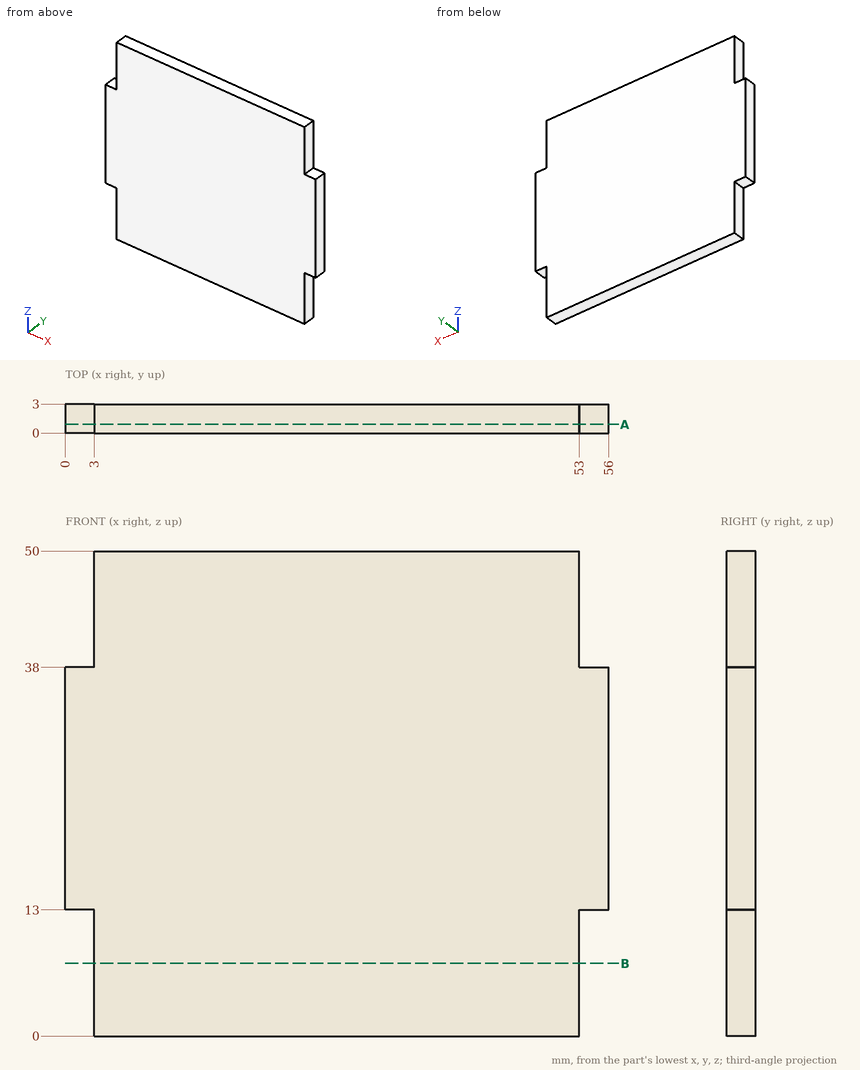
Design review of the part shown in the three views and the two pictorial views. Dimensions are in mm from the part's minimum x, y and z. Give positions to 0.01 mm unless a question says otherwise; leave off trailing zeros. Write each loop counter-clockwise with the first axis right and the second up, starting at its lowest first coordinate (ties: lowest second). Pieces come first, ordered by that corner, then holes.
(1) Clearance check with flat-ended pins moving along their axes: pin 1 Ø1.5 at (y, z) = (1.5, 47) entering from -X; pin 2 Ø1.5 at (y, z) = (1.5, 41) entering from +X; pin 3 Ø0.9 at (x, y) = (1.5, 2) entering from +Z. State where each tip first meets the part, or that it passes through.
Checked values:
pin 1: stops at x = 3
pin 2: stops at x = 53
pin 3: stops at z = 38
(2) Wall thickness on line 1 along X through (y, z) = (1.3, 8): over which ranges is the line inside the solid? List them lowest first.
Checked values:
line 1: x = 3 to 53
(3) Add section B-B (z = 7.5). Give the boundary of the cut face in (x, y).
Checked values:
outline: (3, 0) - (53, 0) - (53, 3) - (3, 3) - close
(4) Add section A-A (y = 0.9). Give the boundary of the cut face in (x, z), and give its area (3 significant figures).
Checked values:
outline: (0, 13) - (3, 13) - (3, 0) - (53, 0) - (53, 13) - (56, 13) - (56, 38) - (53, 38) - (53, 50) - (3, 50) - (3, 38) - (0, 38) - close
area: 2,650 mm2
